```python
from build123d import *

# Parameters (mm, degrees)
SKETCH1_R           = 7.161972439
BOSS_EXTRUDE1_DEPTH = 5.8
CUT_EXTRUDE1_DEPTH  = 12.671662197
CIRPATTERN1_COUNT   = 15
CUT_EXTRUDE2_DEPTH  = 12.659198501


with BuildPart() as part:
    # Sketch1 → Boss-Extrude1 (new body)
    with BuildSketch(Plane(origin=(0, 0, 0), x_dir=(1, 0, 0), z_dir=(0, 1, 0))):
        with Locations(Location((0, 0, 0), (0, 0, 270))):
            Circle(SKETCH1_R)
    extrude(amount=BOSS_EXTRUDE1_DEPTH)

    # Sketch2 → Cut-Extrude1 (cut, through all)
    with BuildSketch(Plane(origin=(0, 5.8, 0), x_dir=(1, 0, 0), z_dir=(0, 1, 0))):
        with BuildLine():
            Line((-0.879885324, 6.559804793), (-0.95, 6.825530337))
            ThreePointArc((-0.95, 6.825530337), (-1.079308013, 7.002279754), (-1.294287054, 7.044052118))
            ThreePointArc((-1.294287054, 7.044052118), (-2.118539526, 6.841464719), (-2.913036628, 6.54278739))
            Line((-2.913036628, 6.54278739), (-2.913036628, 7.161972439))
            Line((-2.913036628, 7.161972439), (2.913036628, 7.161972439))
            Line((2.913036628, 7.161972439), (2.913036628, 6.54278739))
            ThreePointArc((2.913036628, 6.54278739), (2.118539526, 6.841464719), (1.294287054, 7.044052118))
            ThreePointArc((1.294287054, 7.044052118), (1.079308013, 7.002279754), (0.95, 6.825530337))
            Line((0.95, 6.825530337), (0.879885324, 6.559804793))
            ThreePointArc((0.879885324, 6.559804793), (0, 5.881972439), (-0.879885324, 6.559804793))
        make_face()
    cut_extrude1 = extrude(amount=-CUT_EXTRUDE1_DEPTH, mode=Mode.SUBTRACT)

    # CirPattern1: Cut-Extrude1 ×15 about axis
    cirpattern1_axis = Axis((0, 0, 0), (0, 1, 0))
    for i in range(1, CIRPATTERN1_COUNT):
        add(cut_extrude1.rotate(cirpattern1_axis, i * 360 / CIRPATTERN1_COUNT), mode=Mode.SUBTRACT)

    # Sketch3 → Cut-Extrude2 (cut, through all)
    with BuildSketch(Plane.XZ):
        with BuildLine():
            Line((1.84729532, 2.3), (-1.84729532, 2.3))
            ThreePointArc((-1.84729532, 2.3), (0, -2.95), (1.84729532, 2.3))
        make_face()
    extrude(amount=-CUT_EXTRUDE2_DEPTH, mode=Mode.SUBTRACT)


solid = part.part
```
Can you work these out from the model? Positions are in its coordinate system, mm. Coordinates: 2 decimals unless noted, no trailing zeros. Order: outer loops, then holes, each group sorted by start corner. A loop starts at its lowest first (then second) coordinate and runs counter-clockwise, first axis right, second up. Notation, with made-up numbers: (53.25, -7) -> (62.25, -7) arc R10 ccw to (62.25, 0) -> close; hole circle Ø3 at (-38, 72.5). An arc over 180 degrees is marked (long way). Write each question's results on one line, items separated by ' | '.
Item 1: I want a section at B-B, the plane z = 0. Write out the boundary of the cut face in (x, y).
Results are:
outline: (-6.19, 0) -> (-2.95, 0) -> (-2.95, 5.8) -> (-6.19, 5.8) -> close; (2.95, 0) -> (6.19, 0) -> (6.19, 5.8) -> (2.95, 5.8) -> close
Item 2: I'm going to push flat-ended pins straight in: pin 1 Ø3 at (x, y) = (3, 3) entering from -Z; pin 2 Ø1.5 at (y, z) = (1.5, -2.5) entering from +X; pin 3 Ø1.1 at (x, y) = (0, 3.5) entering from -Z. Where does each tip first touch, or does it pass through?
Results are:
pin 1: z = -7 | pin 2: x = 6.34 | pin 3: z = -6.07
Item 3: I want a section at A-A, the plane x = 0. Write out the boundary of the cut face in (y, z).
Results are:
outline: (0, -5.88) -> (5.8, -5.88) -> (5.8, -2.95) -> (0, -2.95) -> close; (0, 2.3) -> (5.8, 2.3) -> (5.8, 7.16) -> (0, 7.16) -> close
Item 4: If I drill on line 1 along Z through (x, y) = (0, 3.9); line 2 along X through (y, z) = (2.9, 0); line 3 along X through (y, z) = (0.35, -0.5), over which ranges is the centre line in solid material (lowest first)?
Results are:
line 1: -5.88 to -2.95, 2.3 to 7.16 | line 2: -6.19 to -2.95, 2.95 to 6.19 | line 3: -7.14 to -2.91, 2.91 to 7.14
Item 5: If we mould it in two halves opening along Z, with no side actions, what happens to faces 1 (the face through (0, 3, 2.3)), 2 (the face through (-5.85, 2.94, 0.6)), 3 (the face through (-3.1, 0, 0)), 4 (the face through (-1.24, 2.94, 5.75))? For each: +Z half, -Z half, draft (parallel to the pull), parting line (faces both ways), or undercut.
Results are:
face 1: undercut | face 2: undercut | face 3: draft | face 4: +Z half
